The listing builds one solid part. Answer for the finished solid, in the listing's coordinates (mm). Face numbers are marked on the shaded views. Coordinates: 2 decimals unless noted, no trailing zeros. Write each loop counter-clockwise with the first axis right and the second up, starting at its lowest first coordinate (ties: lowest second). Pieces come first, ordered by that corner, then holes.
Autodesk Inventor part; units mm, degrees
ref_plane "YZ Plane" through (0, 0, 0) normal (1, 0, 0) x (0, 1, 0)
ref_plane "XZ Plane" through (0, 0, 0) normal (0, 1, 0) x (-1, 0, 0)
ref_plane "XY Plane" through (0, 0, 0) normal (0, 0, 1) x (1, 0, 0)
sketch "Sketch1" plane through (0, 0, 0) normal (1, 0, 0) x (0, 1, 0)
  line L0 (-12.7, 939.8) -> (-12.7, 914.4)
  line L1 (-12.7, 914.4) -> (25.4, 914.4)
  line L2 (25.4, 914.4) -> (25.4, 863.6)
  line L3 (25.4, -914.4) -> (-12.7, -914.4)
  line L4 (-12.7, -914.4) -> (-12.7, -939.8)
  line L5 (-12.7, -939.8) -> (50.8, -939.8)
  line L6 (50.8, -939.8) -> (50.8, -838.2)
  line L7 (50.8, 939.8) -> (-12.7, 939.8)
  line L8 (25.4, 863.6) -> (-25.4, 863.6)
  line L9 (-25.4, 863.6) -> (-25.4, -863.6)
  line L10 (-25.4, -863.6) -> (25.4, -863.6)
  line L11 (25.4, -863.6) -> (25.4, -914.4)
  line L12 (25.4, 863.6) -> (25.4, -863.6) construction
  line L13 (50.8, -838.2) -> (0, -838.2)
  line L14 (0, -838.2) -> (0, 838.2)
  line L15 (0, 838.2) -> (50.8, 838.2)
  line L16 (50.8, 838.2) -> (50.8, 939.8)
  line L17 (50.8, -838.2) -> (50.8, 838.2) construction
  point P0 (0, 0)
  point P1 (0, 0)
  point P2 (0, 0)
  dimension "d4" = 25.4
  dimension "d5" = 1879.6
  dimension "d7" = 63.5
  dimension "d11" = 50.8
  dimension "d12" = 50.8
  dimension "d13" = 50.8
  dimension "d14" = 76.2
  dimension "d15" = 25.4
  dimension "d16" = 25.4
  dimension "d17" = 25.4
extrude "Extrusion1" add sketch "Sketch1" along normal mid plane 914.4
fillet "Fillet1" radius 25.4 4 edges at (0, 50.8, 939.8) (0, 50.8, -939.8) (0, 50.8, -838.2) (0, 50.8, 838.2)
properties part number "Gondola Base Plate" material "Steel, Alloy"
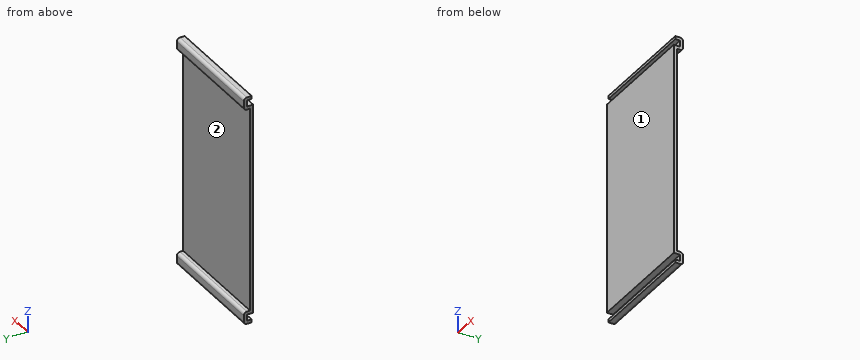
Q1. The part is cut by section B-B, the plane z = -764. Write down the section's boundary in (x, y), then the cut area to 3 significant figures.
Answers below:
outline: (-457.2, -25.4) - (457.2, -25.4) - (457.2, 0) - (-457.2, 0) - close
area: 23,200 mm2
Q2. The part is cut by section A-A, the plane x = 340.5. Write down the section's boundary in (y, z).
Answers below:
outline: (-25.4, -863.6) - (25.4, -863.6) - (25.4, -914.4) - (-12.7, -914.4) - (-12.7, -939.8) - (25.4, -939.8) arc R25.4 ccw to (50.8, -914.4) - (50.8, -863.6) arc R25.4 ccw to (25.4, -838.2) - (0, -838.2) - (0, 838.2) - (25.4, 838.2) arc R25.4 ccw to (50.8, 863.6) - (50.8, 914.4) arc R25.4 ccw to (25.4, 939.8) - (-12.7, 939.8) - (-12.7, 914.4) - (25.4, 914.4) - (25.4, 863.6) - (-25.4, 863.6) - close
Q3. Determine the mould class of the marked faces 1 and 2 for opening direction Z: released by +Z, released by -Z, zero draft, split by the parting line, or undercut.
Answers below:
face 1: zero draft
face 2: undercut
Q4. Find the intervals of material crossed by probe 1 along Z at (x, y) = (-346, 10.5); probe 2 along Z at (x, y) = (98.5, 28.5); probe 3 along Z at (x, y) = (-378, -5), in increasing order.
Answers below:
probe 1: z = -939.8 to -914.4, -863.6 to -838.2, 838.2 to 863.6, 914.4 to 939.8
probe 2: z = -939.61 to -838.39, 838.39 to 939.61
probe 3: z = -939.8 to -914.4, -863.6 to 863.6, 914.4 to 939.8
Q5. Given pin 1 (20.5 mm diameter, centred on x = 179.5, z = 926.5, fed in from -Y); pin 2 (15 mm diameter, centred on x = -101.5, z = 892, fed in from -Y); pin 3 (5 mm diameter, centred on x = 85.5, y = 32.5, fed in from +Z), each flat-ended and moving along its own axis, determine where each tip first touches the part or whether it passes through.
Answers below:
pin 1: stops at y = -12.7
pin 2: stops at y = 25.4
pin 3: stops at z = 939.38
